Part model, mm, in its own coordinate system. A direction names the side the tool comes from. Give positions to 0.01 mm unless a question says otherwise; leave off trailing zeros. Write each loop counter-clockwise with the first axis right and the second up, starting at its lowest first coordinate (ties: lowest second). Pieces come first, ordered by that corner, then holes. Notation, with made-up numbers: M -5.5,17.25 L 43.5,17.25 A31 cw 43.5,56.25 Z; hole C 64.5,1 d7. An arc over 180 degrees is marked long. Use a Markdown table: item, result.
```python
from build123d import *

# Parameters (mm, degrees)
SKETCH_2_W                  = 80
SKETCH_2_H                  = 45
EXTRUDE_2_DEPTH             = 5
HOLE_WIZARD_M3_1_AT_2_COUNT = 2
HOLE_WIZARD_M3_1_AT_2_PITCH = 38
SKETCH_5_R                  = 5
CUT_EXTRUDE_1_DEPTH         = 10
CUT_EXTRUDE_2_DEPTH         = 10


with BuildPart() as part:
    # 草图2 → 凸台-拉伸2 (new body)
    with BuildSketch(Plane(origin=(0, 0, 0), x_dir=(0, 0, -1), z_dir=(1, 0, 0))):
        Rectangle(SKETCH_2_W, SKETCH_2_H)
    extrude(amount=-EXTRUDE_2_DEPTH)

    # 草图12 → M3 螺纹孔1 (revolve, cut)
    with BuildSketch(Plane(origin=(-2.5, 19, 40), x_dir=(0, -1, 0), z_dir=(1, 0, 0))):
        Polygon((0, 0), (0, 8.251075774), (1.25, 7.5), (1.25, 0), align=None)
    hole_wizard_m3_1 = revolve(axis=Axis((-2.5, 19, 46.35), (0, 0, -1)), mode=Mode.SUBTRACT)

    # M3 螺纹孔1 at 2: M3 螺纹孔1 ×2
    with Locations(*[(0, -i * HOLE_WIZARD_M3_1_AT_2_PITCH, 0) for i in range(1, HOLE_WIZARD_M3_1_AT_2_COUNT)]):
        add(hole_wizard_m3_1, mode=Mode.SUBTRACT)

    # 镜向1: M3 螺纹孔1 across plane
    add(hole_wizard_m3_1.mirror(Plane.XY), mode=Mode.SUBTRACT)

    # 镜向1 copy 1 sketch → 镜向1 copy 1 (revolve, cut)
    with BuildSketch(Plane(origin=(-2.5, -19, -40), x_dir=(0, -1, 0), z_dir=(1, 0, 0))):
        Polygon((0, 0), (0, -8.251075774), (1.25, -7.5), (1.25, 0), align=None)
    revolve(axis=Axis((-2.5, -19, -46.35), (0, 0, -1)), mode=Mode.SUBTRACT)

    # 草图5 → 切除-拉伸1 (cut)
    with BuildSketch(Plane(origin=(0, 0, 0), x_dir=(0, 0, -1), z_dir=(1, 0, 0))):
        with Locations((-7, 0)):
            Circle(SKETCH_5_R)
        with Locations((23, 0)):
            Circle(SKETCH_5_R)
        with Locations((-22, 0)):
            Circle(SKETCH_5_R)
    extrude(amount=-CUT_EXTRUDE_1_DEPTH, mode=Mode.SUBTRACT)

    # 草图13 → 切除-拉伸2 (cut)
    with BuildSketch(Plane(origin=(0, 0, 0), x_dir=(0, 0, -1), z_dir=(1, 0, 0))):
        Polygon((-27, 0), (-27, 15), (-13.340798137, 15), (-4.226787528, 15), (-2, 15), (-2, 0), (-12, 0), (-12, 5), (-17, 5), (-17, 0), align=None)
    extrude(amount=-CUT_EXTRUDE_2_DEPTH, mode=Mode.SUBTRACT)


solid = part.part
```
1. Drop a flat-ended pin along its axis: P1, Ø9, axis at y = 0, z = -23, coming from the +X side (1 decimal). Give the stop position or say it passes through.
Findings below:
| item | result |
|---|---|
| P1 | through |
2. Cut at C-C, the plane y = 2. Give the cut face in (x, z), then the cut area to 3 significant figures.
Findings below:
| item | result |
|---|---|
| outline | M -5,-40 L 0,-40 L 0,-27.58 L -5,-27.58 Z; M -5,-18.42 L 0,-18.42 L 0,2 L -5,2 Z; M -5,12 L 0,12 L 0,17 L -5,17 Z; M -5,27 L 0,27 L 0,40 L -5,40 Z |
| area | 254 mm2 |
3. Cut at B-B, the plane y = 14. Give the cut face in (x, z), then the cut area to 3 significant figures.
Findings below:
| item | result |
|---|---|
| outline | M -5,-40 L 0,-40 L 0,2 L -5,2 Z; M -5,27 L 0,27 L 0,40 L -5,40 Z |
| area | 275 mm2 |
4. Tool access for faces 4 (the flat face through (-5, 0, 1)), 5 (the flat face through (-2, 15, 14)), 6 (the cylindrical face through (-2.021, 17.845, 36.302)): list every direction of +Z, -Z, +X, -X, +Y, -Y with a clear straight run to the whole face (end or side of a thin tool).
Findings below:
| item | result |
|---|---|
| face 4 | +Z, -Z, -X, +Y, -Y |
| face 5 | +X, -X |
| face 6 | +Z |
5. Cut at A-A, the plane z = 10. Give the cut face in (x, y).
Findings below:
| item | result |
|---|---|
| outline | M -5,-22.5 L 0,-22.5 L 0,-4 L -5,-4 Z; M -5,15 L 0,15 L 0,22.5 L -5,22.5 Z |
6. Two-plate mould, pull along Y, no slides. Class faces 1 (the flat face through (-2, -22.5, 1)), 2 (the flat face through (-2, 0, 40)), 3 (the cylindrical face through (-2.021, -20.155, -36.302)): released by +Y, released by -Y, zero draft, split by the parting line, or undercut.
Findings below:
| item | result |
|---|---|
| face 1 | released by -Y |
| face 2 | zero draft |
| face 3 | undercut |
7. Drill centre lines: L1, parallel to Y at x = -2.5, z = -37; L2, parallel to Z at x = -3, y = 13.5; L3, parallel to Y at x = -4.2, z = 16. Where is each one in solid material? Low to high.
Findings below:
| item | result |
|---|---|
| L1 | -22.5 to -20.25, -17.75 to 17.75, 20.25 to 22.5 |
| L2 | -40 to 2, 27 to 40 |
| L3 | -22.5 to 5, 15 to 22.5 |
